Design review of the part built by this model. Coordinates are the model's own, in mm. A direction names the side the tool comes from. Coordinates: 2 decimals unless noted, no trailing zeros. Write each loop counter-clockwise with the first axis right and the second up, starting at its lowest first coordinate (ties: lowest second). Pieces come first, ordered by that corner, then holes. Notation, with made-up numbers: (13, 1) - (26, 1) arc R19 cw to (26, 18) - close; hole circle Ø1 at (2.25, 86). An arc over 180 degrees is marked (long way). Use a Markdown table: item, result.
from build123d import *

# Parameters (mm, degrees)
SKETCH_1_W          = 19
SKETCH_1_H          = 35
SKETCH_1_R          = 1.5
EXTRUDE_1_DEPTH     = 3
SKETCH_2_W          = 9.5
SKETCH_2_H          = 19.5
EXTRUDE_2_DEPTH     = 16
SKETCH_3_R          = 4.05
CUT_EXTRUDE_1_DEPTH = 16
SKETCH_4_W          = 3
SKETCH_4_H          = 19.5
CUT_EXTRUDE_2_DEPTH = 16
FILLET_1_R          = 2
SKETCH_5_R          = 5
CUT_EXTRUDE_3_DEPTH = 6
FILLET_3_R          = 4


with BuildPart() as part:
    # 草图1 → 凸台-拉伸1 (new body)
    with BuildSketch(Plane.XY):
        Rectangle(SKETCH_1_W, SKETCH_1_H)
        with Locations((-6, 14)):
            Circle(SKETCH_1_R, mode=Mode.SUBTRACT)
        with Locations((6, 14)):
            Circle(SKETCH_1_R, mode=Mode.SUBTRACT)
        with Locations((6, -14)):
            Circle(SKETCH_1_R, mode=Mode.SUBTRACT)
        with Locations((-6, -14)):
            Circle(SKETCH_1_R, mode=Mode.SUBTRACT)
    extrude(amount=EXTRUDE_1_DEPTH)

    # 草图2 → 凸台-拉伸2 (add)
    with BuildSketch(Plane.XY.offset(3)):
        Rectangle(SKETCH_2_W, SKETCH_2_H)
    extrude(amount=EXTRUDE_2_DEPTH)

    # 草图3 → 切除-拉伸1 (cut)
    with BuildSketch(Plane.ZY.offset(4.75)):
        with Locations(Location((14, 0, 0), (0, 0, 270))):
            Circle(SKETCH_3_R)
    extrude(amount=-CUT_EXTRUDE_1_DEPTH, mode=Mode.SUBTRACT)

    # 草图4 → 切除-拉伸2 (cut)
    with BuildSketch(Plane.ZY.offset(4.75)):
        with Locations((17.5, 0)):
            Rectangle(SKETCH_4_W, SKETCH_4_H)
    extrude(amount=-CUT_EXTRUDE_2_DEPTH, mode=Mode.SUBTRACT)

    # 圆角1
    fillet_1_edges = [part.edges().sort_by_distance(p)[0] for p in [
        (9.5, -17.5, 1.5),
        (-9.5, -17.5, 1.5),
        (-9.5, 17.5, 1.5),
        (9.5, 17.5, 1.5),
    ]]
    fillet(fillet_1_edges, radius=FILLET_1_R)

    # 草图5 → 切除-拉伸3 (cut)
    with BuildSketch(Plane(origin=(0, 0, 0), x_dir=(-1, 0, 0), z_dir=(0, 0, -1))):
        Circle(SKETCH_5_R)
    extrude(amount=-CUT_EXTRUDE_3_DEPTH, mode=Mode.SUBTRACT)

    # 圆角3
    fillet_3_edges = [part.edges().sort_by_distance(p)[0] for p in [
        (0, 9.75, 16),
        (0, -9.75, 16),
    ]]
    fillet(fillet_3_edges, radius=FILLET_3_R)


solid = part.part
(1) For L1, parallel to Y at x = -6, z = 1.1; L2, parallel to Y at x = 0, z = 1.95; L3, parallel to Z at x = -0.75, y = -15, list the stretches that pass through material, from the lowest coordinate up. Write a range as from..to.
Determined:
| item | result |
|---|---|
| L1 | -17.5..-15.5, -12.5..12.5, 15.5..17.5 |
| L2 | -17.5..-5, 5..17.5 |
| L3 | 0..3 |
(2) For pin 1 (2.5 mm diameter, centred on x = 6, y = 14, fed in from +Z); pin 2 (1 mm diameter, centred on y = -6, z = 10.5, fed in from -X); pin 3 (3.5 mm diameter, centred on x = 6, y = -14, fed in from +Z); pin 4 (5 mm diameter, centred on x = 7, z = 14, fed in from -Y), all flat-tipped, find the tip position at first contact; note any pin that passes through.
Determined:
| item | result |
|---|---|
| pin 1 | through |
| pin 2 | x = -4.75 |
| pin 3 | z = 3 |
| pin 4 | y = -9.65 |
(3) Take a section at D-D on x = 0. Write out the cut boundary in (y, z), and give its area (3 significant figures).
Determined:
| item | result |
|---|---|
| outline | (-17.5, 0) - (-5, 0) - (-5, 6) - (5, 6) - (5, 0) - (17.5, 0) - (17.5, 3) - (9.75, 3) - (9.75, 12) arc R4 ccw to (5.75, 16) - (3.52, 16) arc R4.05 cw (long way) to (-3.52, 16) - (-5.75, 16) arc R4 ccw to (-9.75, 12) - (-9.75, 3) - (-17.5, 3) - close |
| area | 250 mm2 |
(4) Take a section at B-B on x = -6. Write out the cut boundary in (y, z).
Determined:
| item | result |
|---|---|
| outline | (-17.5, 0) - (-15.5, 0) - (-15.5, 3) - (-17.5, 3) - close; (-12.5, 0) - (12.5, 0) - (12.5, 3) - (-12.5, 3) - close; (15.5, 0) - (17.5, 0) - (17.5, 3) - (15.5, 3) - close |
(5) Take a section at C-C on z = 11. Write out the cut boundary in (x, y), and give its area (3 significant figures).
Determined:
| item | result |
|---|---|
| outline | (-4.75, -9.75) - (4.75, -9.75) - (4.75, -2.72) - (-4.75, -2.72) - close; (-4.75, 2.72) - (4.75, 2.72) - (4.75, 9.75) - (-4.75, 9.75) - close |
| area | 134 mm2 |
(6) Take a section at A-A on y = 14. Write out the cut boundary in (x, z), and give its area (3 significant figures).
Determined:
| item | result |
|---|---|
| outline | (-9.5, 0) - (-7.5, 0) - (-7.5, 3) - (-9.5, 3) - close; (-4.5, 0) - (4.5, 0) - (4.5, 3) - (-4.5, 3) - close; (7.5, 0) - (9.5, 0) - (9.5, 3) - (7.5, 3) - close |
| area | 39.0 mm2 |
(7) Draft analysis for pull direction Z (two halves, no side actions). For faces 1 (the cylindrical face through (-0.07, 0.12, 9.95)), 2 (the flat face through (-4, 4, 0)), 3 (the cylindrical face through (-7.2, 13.1, 1.5)), state which applies: +Z half, -Z half, draft (parallel to the pull), parting line (faces both ways), or undercut.
Determined:
| item | result |
|---|---|
| face 1 | undercut |
| face 2 | -Z half |
| face 3 | draft |
(8) Machinability: for faces 4 (the flat face through (-4.75, 0, 9)), 5 (the cylindrical face through (1.08, -4.88, 2.96)), 6 (the flat face through (0, 9.75, 7)), which of the approach directions +Z, -Z, +X, -X, +Y, -Y give a long, thin tool a straight path to every point of the face, cutting with its end or side? Answer none if there is none.
Determined:
| item | result |
|---|---|
| face 4 | +Z, -X, +Y, -Y |
| face 5 | -Z |
| face 6 | +Z, +X, -X, +Y |
